The drawing under review shows one solid part. Ordinate dimensions are in mm from its lowest x, y, z. Round coordinates to 2 decimals unless told otherwise and drop trailing zeros. Order: outer loops, then holes, each group sorted by start corner. A loop starts at its lowest first (then second) coordinate and runs counter-clockwise, first axis right, second up.
1) Consider section C-C (y = 0.9). Give the number of separate pieces and of enclosed holes in the cut face, then the cut area to 3 significant figures.
2) Consider section D-D (z = 81.5). Give the boundary of the cut face in (x, y) (1 decimal).
3) Clearance check with flat-ended pins moving along their axes: P1, Ø1.3, axis at x = 97.5, y = 1.5, coming from the +Z side (1 decimal); P2, Ø1.5, axis at y = 1.5, z = 134, coming from the -X side; P3, Ø0.8, axis at x = 70.5, y = 1, coming from the -Z side; P4, Ø15, axis at x = 17.43, z = 86.93, coming from the -Y side. State where each tip first meets the part, or that it passes through.
4) Consider section B-B (x = 122). Give the boundary of the cut face in (y, z) (1 decimal).
5) Consider section A-A (z = 129). Give the boundary of the cut face in (x, y) (1 decimal), then the cut area to 3 significant figures.
6) To check wall thickness, follow L1, parallel to X at y = 2.45, z = 43 (1 decimal); L2, parallel to Z at x = 106, y = 2.3 (1 decimal); L3, parallel to X at y = 1.65, z = 148 (1 decimal). State the ranges of each line that lie inside material, in increasing order.
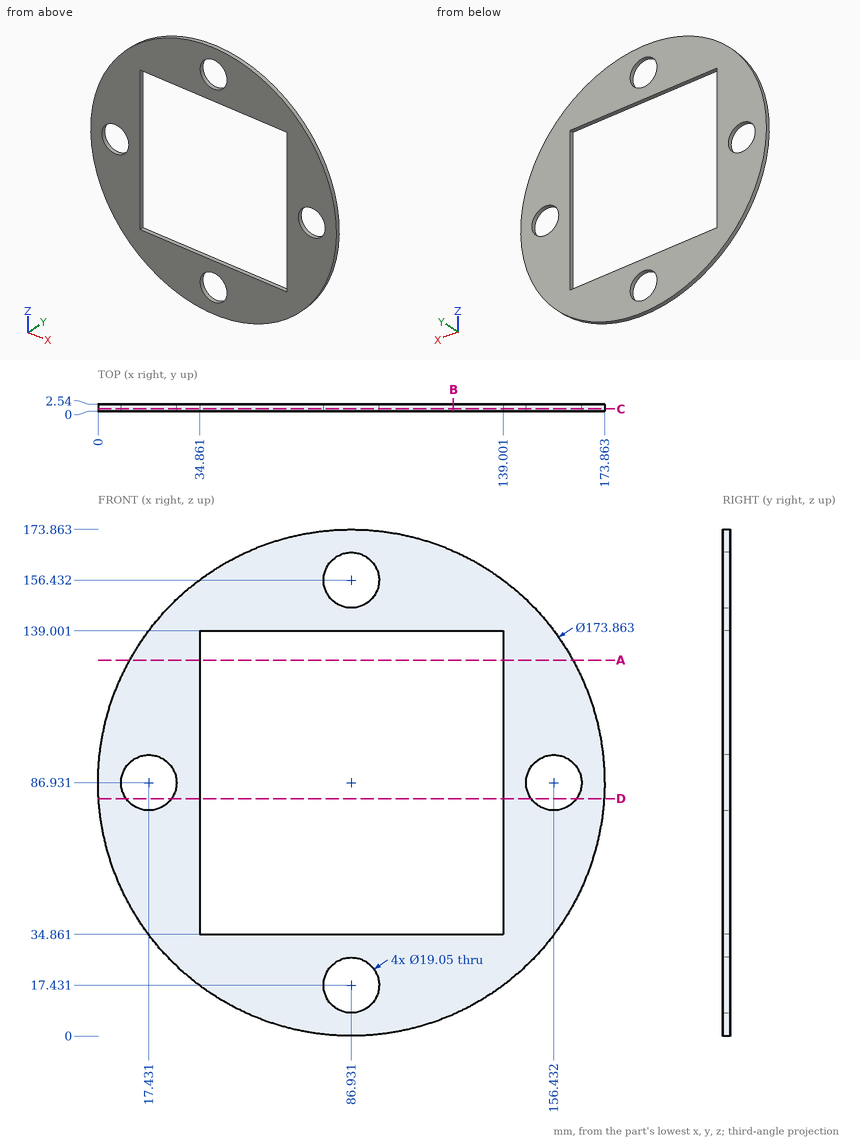
Answer below:
1. separate pieces: 1
1. enclosed holes: 5
1. area: 11,800 mm2
2. outline: (0.2, 0) - (9.6, 0) - (9.6, 2.5) - (0.2, 2.5) - close; (25.3, 0) - (34.9, 0) - (34.9, 2.5) - (25.3, 2.5) - close; (139, 0) - (148.6, 0) - (148.6, 2.5) - (139, 2.5) - close; (164.3, 0) - (173.7, 0) - (173.7, 2.5) - (164.3, 2.5) - close
3. P1: stops at z = 173.3
3. P2: stops at x = 13.37
3. P3: stops at z = 1.49
3. P4: passes through
4. outline: (0, 7.4) - (2.5, 7.4) - (2.5, 34.9) - (0, 34.9) - close; (0, 139) - (2.5, 139) - (2.5, 166.5) - (0, 166.5) - close
5. outline: (10.9, 0) - (34.9, 0) - (34.9, 2.5) - (10.9, 2.5) - close; (139, 0) - (163, 0) - (163, 2.5) - (139, 2.5) - close
5. area: 122 mm2
6. L1: x = 11.9 to 34.9, 139 to 161.9
6. L2: z = 2.1 to 34.9, 139 to 171.7
6. L3: x = 25.1 to 82.5, 91.4 to 148.8
